CAD build for the part. Positions are in the model's coordinates, mm. Face numbers are marked on the shaded views. A direction names the side the tool comes from. Give positions to 0.01 mm unless a question says otherwise; leave off trailing zeros. Loops run counter-clockwise (first coordinate to the right, second up) from the corner with the lowest first, then second, coordinate; pieces in that order, holes last. Notation, with made-up numbers: M 64,5 L 68,5 A11 cw 68,20 Z; hole C 65,60.25 d11. An arc over 180 degrees is marked long. One line per question, with ' | ' between items.
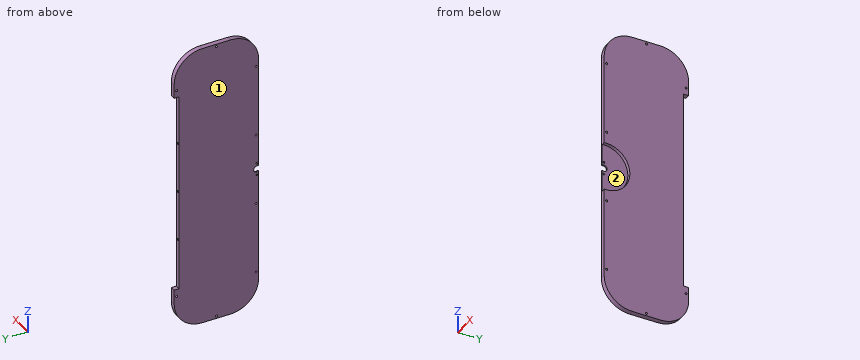
```python
from build123d import *

# Parameters (mm, degrees)
BOSS_EXTRUDE1_DEPTH     = 7
CUT_EXTRUDE1_DEPTH      = 234.343095034
CUT_EXTRUDE1_DEPTH_BACK = 234.343095034
SKETCH2_R               = 1.5
SKETCH2_W               = 280
SKETCH2_H               = 7
CUT_EXTRUDE2_DEPTH      = 230.821669997
CUT_EXTRUDE2_DEPTH_BACK = 10
CUT_EXTRUDE2_START      = 3
SKETCH3_R               = 1.5
SKETCH4_R               = 1.25
CUT_EXTRUDE3_DEPTH      = 10
CUT_EXTRUDE4_DEPTH      = 4
SKETCH6_R               = 4.5
CUT_EXTRUDE5_DEPTH      = 234.272372989
SKETCH7_R               = 34
CUT_EXTRUDE6_DEPTH      = 5


with BuildPart() as part:
    # Sketch1 → Boss-Extrude1 (new body)
    with BuildSketch(Plane(origin=(0, 0, 0), x_dir=(0, 0, -1), z_dir=(1, 0, 0))):
        with BuildLine():
            Line((160, 0), (-160, 0))
            ThreePointArc((-160, 0), (-188.284271247, 11.715728753), (-200, 40))
            Line((-200, 40), (-200, 80))
            ThreePointArc((-200, 80), (-188.284271247, 108.284271247), (-160, 120))
            Line((-160, 120), (160, 120))
            ThreePointArc((160, 120), (188.284271247, 108.284271247), (200, 80))
            Line((200, 80), (200, 40))
            ThreePointArc((200, 40), (188.284271247, 11.715728753), (160, 0))
        make_face()
    extrude(amount=BOSS_EXTRUDE1_DEPTH)

    # Sketch2 → Cut-Extrude1 (cut, two sides: drawn at the far end of the back side and taken through both)
    with BuildSketch(Plane(origin=(7, 0, 0), x_dir=(0, 0, -1), z_dir=(1, 0, 0)).offset(-CUT_EXTRUDE1_DEPTH_BACK)):
        with Locations((-150, 116.5)):
            Circle(SKETCH2_R)
        with Locations((-196.5, 60)):
            Circle(SKETCH2_R)
        with Locations((-50, 3.5)):
            Circle(SKETCH2_R)
        with Locations((-150, 3.5)):
            Circle(SKETCH2_R)
        with Locations(Location((50, 3.5, 0), (0, 0, 180))):
            Circle(SKETCH2_R)
        with Locations(Location((150, 3.5, 0), (0, 0, 180))):
            Circle(SKETCH2_R)
        with Locations(Location((196.5, 60, 0), (0, 0, 180))):
            Circle(SKETCH2_R)
        with Locations(Location((150, 116.5, 0), (0, 0, 180))):
            Circle(SKETCH2_R)
        with Locations((0, 116.5)):
            Rectangle(SKETCH2_W, SKETCH2_H)
    extrude(amount=CUT_EXTRUDE1_DEPTH + CUT_EXTRUDE1_DEPTH_BACK, mode=Mode.SUBTRACT)

    # Sketch3 → Cut-Extrude2 (cut, two sides: drawn at the far end of the back side and taken through both)
    with BuildSketch(Plane(origin=(0, 113, 0), x_dir=(1, 0, 0), z_dir=(0, 1, 0)).offset(CUT_EXTRUDE2_START - CUT_EXTRUDE2_DEPTH_BACK)):
        with Locations(Location((3.5, 70, 0), (0, 0, 90))):
            Circle(SKETCH3_R)
        with Locations(Location((3.5, 0, 0), (0, 0, 90))):
            Circle(SKETCH3_R)
        with Locations(Location((3.5, -70, 0), (0, 0, 90))):
            Circle(SKETCH3_R)
    extrude(amount=CUT_EXTRUDE2_DEPTH + CUT_EXTRUDE2_DEPTH_BACK, mode=Mode.SUBTRACT)

    # Sketch4 → Cut-Extrude3 (cut)
    with BuildSketch(Plane(origin=(7, 0, 0), x_dir=(0, 0, -1), z_dir=(1, 0, 0))):
        with Locations((-8.5, 2.5)):
            Circle(SKETCH4_R)
        with Locations((8.5, 2.5)):
            Circle(SKETCH4_R)
    extrude(amount=-CUT_EXTRUDE3_DEPTH, mode=Mode.SUBTRACT)

    # Sketch5 → Cut-Extrude4 (cut)
    with BuildSketch(Plane(origin=(7, 0, 0), x_dir=(0, 0, -1), z_dir=(1, 0, 0))):
        with BuildLine():
            Line((14, -15), (-14, -15))
            Line((-14, -15), (-14, 5))
            ThreePointArc((-14, 5), (0, 19), (14, 5))
            Line((14, 5), (14, -15))
        make_face()
    extrude(amount=-CUT_EXTRUDE4_DEPTH, mode=Mode.SUBTRACT)

    # Sketch6 → Cut-Extrude5 (cut, through all)
    with BuildSketch(Plane(origin=(3, 0, 0), x_dir=(0, 0, -1), z_dir=(1, 0, 0))):
        with Locations((0, 2.5)):
            Circle(SKETCH6_R)
    extrude(amount=-CUT_EXTRUDE5_DEPTH, mode=Mode.SUBTRACT)

    # Sketch7 → Cut-Extrude6 (cut)
    with BuildSketch(Plane(origin=(7, 0, 0), x_dir=(0, 0, -1), z_dir=(1, 0, 0))):
        with Locations((0, 2.5)):
            Circle(SKETCH7_R)
    extrude(amount=-CUT_EXTRUDE6_DEPTH, mode=Mode.SUBTRACT)


solid = part.part
```
Item 1: Drop flat-ended pins along their axis: P1, Ø4, axis at x = 6, y = 14.5, coming from the -Z side; P2, Ø4, axis at y = 2.5, z = 8.5, coming from the +X side; P3, Ø0.9, axis at x = 3, z = -70.5, coming from the +Y side. Give the stop position or say it passes through.
Conclusion:
P1: z = -192.37 | P2: x = 2 | P3: y = 106
Item 2: 3-axis set-ups, long thin cutter, end or side, ignore diameter. For the marked faces 1 and 2: which of +Z, -Z, +X, -X, +Y, -Y reach the whole face in a straight line?
Conclusion:
face 1: +Z, -Z, -X, +Y, -Y | face 2: +X, -Y
Item 3: Drill centre lines: line 1 along Y through (x, z) = (2.5, -50); line 2 along Y through (x, z) = (4.25, 150); line 3 along Z through (x, y) = (5.25, 116.5). Where is each one in solid material? Low to high. Write a range as [from, to].
Conclusion:
line 1: [0, 2], [5, 113] | line 2: [0, 2], [5, 115], [118, 120] | line 3: [-176.36, -151.5], [-148.5, -140], [140, 148.5], [151.5, 176.36]
Item 4: Saw through at A-A on z = 116.5. Give the cut face in (x, y), and give its area (3 significant figures).
Conclusion:
outline: M 0,0 L 7,0 L 7,113 L 0,113 Z | area: 791 mm²
